from build123d import *

# Parameters (mm, degrees)
BOTTOM_DEPTH       = 5
WALL_W             = 100
WALL_H             = 140
WALL_W_2           = 89.5
WALL_H_2           = 129.5
WALLS_DEPTH        = 30
MAINFILLET_R       = 5
DRILLHOLES_R       = 2
DRILLING_DEPTH     = 45
GASKET_DEPTH       = 2
SKETCH1_R          = 4.75
CUT_EXTRUDE1_DEPTH = 10
IO_HOLES_R         = 4.75
CUT_EXTRUDE2_DEPTH = 70
SKETCH2_R          = 2.5
CUT_EXTRUDE3_DEPTH = 10


with BuildPart() as part:
    # Base → Bottom (new body)
    with BuildSketch(Plane(origin=(0, 0, 0), x_dir=(1, 0, 0), z_dir=(0, 1, 0))):
        Polygon((-50, -70), (-50, 70), (-50, 85), (50, 85), (50, 70), (50, -70), (50, -85), (-50, -85), align=None)
    extrude(amount=-BOTTOM_DEPTH)

    # Wall → Walls (add)
    with BuildSketch(Plane(origin=(0, 0, 0), x_dir=(1, 0, 0), z_dir=(0, 1, 0))):
        Rectangle(WALL_W, WALL_H)
        Rectangle(WALL_W_2, WALL_H_2, mode=Mode.SUBTRACT)
        with BuildLine():
            Line((-44.75, -57.3), (-44.75, -64.75))
            Line((-44.75, -64.75), (-37.3, -64.75))
            ThreePointArc((-37.3, -64.75), (-39.48205448, -59.48205448), (-44.75, -57.3))
        make_face()
        with BuildLine():
            ThreePointArc((44.75, -57.3), (39.48205448, -59.48205448), (37.3, -64.75))
            Line((37.3, -64.75), (44.75, -64.75))
            Line((44.75, -64.75), (44.75, -57.3))
        make_face()
        with BuildLine():
            Line((-44.75, 64.75), (-44.75, 57.3))
            ThreePointArc((-44.75, 57.3), (-39.48205448, 59.48205448), (-37.3, 64.75))
            Line((-37.3, 64.75), (-44.75, 64.75))
        make_face()
        with BuildLine():
            Line((44.75, 64.75), (37.3, 64.75))
            ThreePointArc((37.3, 64.75), (39.48205448, 59.48205448), (44.75, 57.3))
            Line((44.75, 57.3), (44.75, 64.75))
        make_face()
    extrude(amount=WALLS_DEPTH)

    # MainFillet
    mainfillet_edges = [part.edges().sort_by_distance(p)[0] for p in [
        (-50, -2.5, 85),
        (-50, -2.5, -85),
        (50, -2.5, -85),
        (50, -2.5, 85),
        (-50, 15, 70),
        (50, 15, 70),
        (50, 15, -70),
        (-50, 15, -70),
    ]]
    fillet(mainfillet_edges, radius=MAINFILLET_R)

    # DrillHoles → Drilling (cut)
    with BuildSketch(Plane(origin=(0, 30, 0), x_dir=(-1, 0, 0), z_dir=(0, -1, 0))):
        with Locations((43.612901731, 63.104701387)):
            Circle(DRILLHOLES_R)
        with Locations((43.612901731, -63.104701387)):
            Circle(DRILLHOLES_R)
        with Locations((-43.612901731, -63.104701387)):
            Circle(DRILLHOLES_R)
        with Locations((-43.612901731, 63.104701387)):
            Circle(DRILLHOLES_R)
    extrude(amount=DRILLING_DEPTH, mode=Mode.SUBTRACT)

    # GasketInsert → Gasket (add)
    with BuildSketch(Plane(origin=(0, 30, 0), x_dir=(1, 0, 0), z_dir=(0, 1, 0))):
        with BuildLine():
            Line((-45.95, -58.5), (-45.95, 58.5))
            ThreePointArc((-45.95, 58.5), (-40.249861113, 60.249861113), (-38.5, 65.95))
            Line((-38.5, 65.95), (38.5, 65.95))
            ThreePointArc((38.5, 65.95), (40.249861113, 60.249861113), (45.95, 58.5))
            Line((45.95, 58.5), (45.95, -58.5))
            ThreePointArc((45.95, -58.5), (40.249861113, -60.249861113), (38.5, -65.95))
            Line((38.5, -65.95), (-38.5, -65.95))
            ThreePointArc((-38.5, -65.95), (-40.249861113, -60.249861113), (-45.95, -58.5))
        make_face()
        with BuildLine():
            Line((-37.3, -64.75), (37.3, -64.75))
            ThreePointArc((37.3, -64.75), (39.48205448, -59.48205448), (44.75, -57.3))
            Line((44.75, -57.3), (44.75, 57.3))
            ThreePointArc((44.75, 57.3), (39.48205448, 59.48205448), (37.3, 64.75))
            Line((37.3, 64.75), (-37.3, 64.75))
            ThreePointArc((-37.3, 64.75), (-39.48205448, 59.48205448), (-44.75, 57.3))
            Line((-44.75, 57.3), (-44.75, -57.3))
            ThreePointArc((-44.75, -57.3), (-39.48205448, -59.48205448), (-37.3, -64.75))
        make_face(mode=Mode.SUBTRACT)
    extrude(amount=GASKET_DEPTH)

    # Sketch1 → Cut-Extrude1 (cut)
    with BuildSketch(Plane.XY.offset(70)):
        with Locations((0, 15)):
            Circle(SKETCH1_R)
    extrude(amount=-CUT_EXTRUDE1_DEPTH, mode=Mode.SUBTRACT)

    # IO Holes → Cut-Extrude2 (cut)
    with BuildSketch(Plane.XY):
        with Locations((-22.5, 15)):
            Circle(IO_HOLES_R)
        with Locations((22.5, 15)):
            Circle(IO_HOLES_R)
    extrude(amount=-CUT_EXTRUDE2_DEPTH, mode=Mode.SUBTRACT)

    # Sketch2 → Cut-Extrude3 (cut)
    with BuildSketch(Plane(origin=(0, 0, 0), x_dir=(1, 0, 0), z_dir=(0, 1, 0))):
        with Locations((0, 77.5)):
            Circle(SKETCH2_R)
        with Locations((0, -77.5)):
            Circle(SKETCH2_R)
    extrude(amount=-CUT_EXTRUDE3_DEPTH, mode=Mode.SUBTRACT)


solid = part.part
Source: CAD feature listing. Evaluate the final solid. Frame: model axes, mm. A direction names the side the tool comes from. Round coordinates to 2 decimals unless told otherwise and drop trailing zeros. Order: outer loops, then holes, each group sorted by start corner. A loop starts at its lowest first (then second) coordinate and runs counter-clockwise, first axis right, second up. Notation, with made-up numbers: (-31.75, 22.25) - (-24.75, 22.25) arc R13 ccw to (-24.75, 41.25) - close; hole circle Ø8 at (27.25, 55.5). An arc over 180 degrees is marked (long way). Use a Markdown table: item, result. Add a question column.
1. Set-up query: faces 4 (the cylindrical face through (-0.62, 19.71, 67.41)), 5 (the cylindrical face through (-17.97, 16.43, -67.34)), 6 (the flat face through (44.75, 16, 1)), 7 (the cylindrical face through (49, 15, 68)). Return all of +Z, -Z, +X, -X, +Y, -Y with unobstructed straight access to the full face (end or side cutting, diameter ignored); none if empty.
2. Section query C-C (y = 15). Give the number of separate pieces and of enclosed holes in the cut face, then the cut area to 3 significant figures.
3. Mould query, pull axis Z, two halves, no side actions, for faces 1 (the cylindrical face through (27.03, 16.43, -67.34)), 2 (the flat face through (-44.75, 16, -1)), 3 (the flat face through (-1, 15, -70)). Classes: +Z half, -Z half, draft (parallel to the pull), parting line (faces both ways), or undercut.
4. Section query A-A (z = -77.5). Return the cut outline in (x, y).
5. Section query B-B (x = 0). Return the cut outline in (y, z), then the cut area to 3 significant figures.
6. Line query: probe 1 along Z at (x, y) = (13.5, 0.5); probe 2 along Y at (x, z) = (22, -68); probe 3 along X at (y, z) = (28.5, -37.5). Output: solid intervals per line, ascending.
7. Section query D-D (x = -22.5). Return the cut outline in (y, z), then the cut area to 3 significant figures.
8. First-contact query: pin 1 (1.6 mm diameter, centred on y = 31, z = -16.5, fed in from -X); pin 2 (10 mm diameter, centred on x = 2.5, y = 25.5, fed in from -Z); pin 3 (10 mm diameter, centred on x = -16, z = -76.5, fed in from +Y). Flat tips, straight axial feed; report the tip coordinate or a pass-through.
Derived:
| question | item | result |
|---|---|---|
| 1 | face 4 | +Z |
| 1 | face 5 | -Z |
| 1 | face 6 | +Y |
| 1 | face 7 | +Z, +X, +Y |
| 2 | separate pieces | 3 |
| 2 | enclosed holes | 4 |
| 2 | area | 2,360 mm2 |
| 3 | face 1 | draft |
| 3 | face 2 | undercut |
| 3 | face 3 | -Z half |
| 4 | outline | (-50, -5) - (-2.5, -5) - (-2.5, 0) - (-50, 0) - close; (2.5, -5) - (50, -5) - (50, 0) - (2.5, 0) - close |
| 5 | outline | (-5, -85) - (0, -85) - (0, -80) - (-5, -80) - close; (-5, -75) - (0, -75) - (0, -70) - (30, -70) - (30, -65.95) - (32, -65.95) - (32, -64.75) - (0, -64.75) - (0, 64.75) - (10.25, 64.75) - (10.25, 70) - (0, 70) - (0, 75) - (-5, 75) - close; (-5, 80) - (0, 80) - (0, 85) - (-5, 85) - close; (19.75, 64.75) - (32, 64.75) - (32, 65.95) - (30, 65.95) - (30, 70) - (19.75, 70) - close |
| 5 | area | 1,070 mm2 |
| 6 | probe 1 | -70 to -64.75, 64.75 to 70 |
| 6 | probe 2 | -5 to 10.28, 19.72 to 30 |
| 6 | probe 3 | -50 to -44.75, 44.75 to 50 |
| 7 | outline | (-5, -85) - (0, -85) - (0, -70) - (10.25, -70) - (10.25, -64.75) - (0, -64.75) - (0, 64.75) - (32, 64.75) - (32, 65.95) - (30, 65.95) - (30, 70) - (0, 70) - (0, 85) - (-5, 85) - close; (19.75, -70) - (30, -70) - (30, -65.95) - (32, -65.95) - (32, -64.75) - (19.75, -64.75) - close |
| 7 | area | 1,120 mm2 |
| 8 | pin 1 | x = -45.95 |
| 8 | pin 2 | z = -70 |
| 8 | pin 3 | y = 0 |
